Geometry check sheet. Reference: the model listing, model coordinates, mm. Face numbers are marked on the shaded views. A direction names the side the tool comes from. Round coordinates to 2 decimals unless told otherwise and drop trailing zeros. Loops run counter-clockwise (first coordinate to the right, second up) from the corner with the lowest first, then second, coordinate; pieces in that order, holes last. Notation, with made-up numbers: (11, 39) -> (47, 39) arc R24 ccw to (47, 77) -> close; hole circle Ø5 at (72, 63). An arc over 180 degrees is marked (long way). Use a Markdown table: item, result. Add a question column.
Q1. Sectioned sample at A-A, the plane x = 0. Enter the section's corners in (y, z), then the cut area to 3 significant figures.
Q2. Gauge pin test, flat ends, axial feed: P1, Ø2, axis at y = 35, z = 11.5, coming from the +X side; P2, Ø6, axis at x = 20, y = 0, coming from the +Z side; P3, Ø6, axis at y = -29, z = 10, coming from the +X side; P4, Ø3, axis at x = -20, y = 0, coming from the -Z side. Record the tip position at first contact, or that the pin passes through.
Q3. Material ranges on L1, parallel to Y at x = 0, z = 16; L2, parallel to Y at x = 0, z = 3.5; L3, parallel to Y at x = -1, z = 25.5, recorded low to high.
Q4. Sectioned sample at C-C, the plane y = 40. Enter the section's corners in (x, z), then the cut area to 4 significant figures.
Q5. Release check for a two-part mould opening along X. For the marked faces 3, 4 and 5 record: released by +X, released by -X, zero draft, split by the parting line, or undercut.
Q6. Sectioned sample at B-B, the plane y = 0. Enter the section's corners in (x, z), then the cut area to 3 significant figures.
Q7. Set-up check for the marked faces 1 and 2: record each of +Z, -Z, +X, -X, +Y, -Y from which the full face is reachable in a straight line by a thin tool's end or side.
Q8. Sectioned sample at D-D, the plane x = 20. Enter the section's corners in (y, z), then the cut area to 3 significant figures.
```python
from build123d import *

# Parameters (mm, degrees)
SKETCH1_R           = 50
SKETCH1_R_2         = 16
BOSS_EXTRUDE1_DEPTH = 8
SKETCH2_R           = 50
SKETCH2_R_2         = 30
BOSS_EXTRUDE2_DEPTH = 37
SKETCH3_R           = 2.5
CUT_EXTRUDE1_DEPTH  = 46
SKETCH4_R           = 2.5
CUT_EXTRUDE2_DEPTH  = 9


with BuildPart() as part:
    # Sketch1 → Boss-Extrude1 (new body)
    with BuildSketch(Plane.XY):
        Circle(SKETCH1_R)
        Circle(SKETCH1_R_2, mode=Mode.SUBTRACT)
    extrude(amount=BOSS_EXTRUDE1_DEPTH)

    # Sketch2 → Boss-Extrude2 (add)
    with BuildSketch(Plane.XY.offset(8)):
        Circle(SKETCH2_R)
        Circle(SKETCH2_R_2, mode=Mode.SUBTRACT)
    extrude(amount=BOSS_EXTRUDE2_DEPTH)

    # Sketch3 → Cut-Extrude1 (cut, through all)
    with BuildSketch(Plane.XY.offset(45)):
        with Locations((0, 40)):
            Circle(SKETCH3_R)
        with Locations((34.641016151, -20)):
            Circle(SKETCH3_R)
        with Locations((-34.641016151, -20)):
            Circle(SKETCH3_R)
    extrude(amount=-CUT_EXTRUDE1_DEPTH, mode=Mode.SUBTRACT)

    # Sketch4 → Cut-Extrude2 (cut, through all)
    with BuildSketch(Plane.XY.offset(8)):
        with Locations((0, 20)):
            Circle(SKETCH4_R)
        with Locations((20, 0)):
            Circle(SKETCH4_R)
        with Locations((0, -20)):
            Circle(SKETCH4_R)
        with Locations((-20, 0)):
            Circle(SKETCH4_R)
    extrude(amount=-CUT_EXTRUDE2_DEPTH, mode=Mode.SUBTRACT)


solid = part.part
```
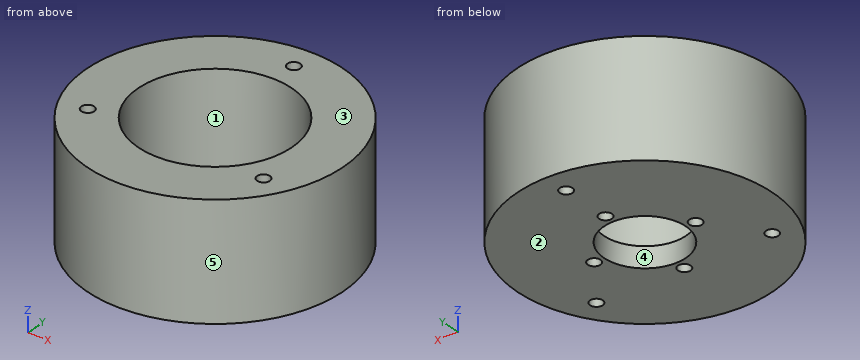
Values:
| question | item | result |
|---|---|---|
| 1 | outline | (-50, 0) -> (-22.5, 0) -> (-22.5, 8) -> (-30, 8) -> (-30, 45) -> (-50, 45) -> close; (-17.5, 0) -> (-16, 0) -> (-16, 8) -> (-17.5, 8) -> close; (16, 0) -> (17.5, 0) -> (17.5, 8) -> (16, 8) -> close; (22.5, 0) -> (37.5, 0) -> (37.5, 45) -> (30, 45) -> (30, 8) -> (22.5, 8) -> close; (42.5, 0) -> (50, 0) -> (50, 45) -> (42.5, 45) -> close |
| 1 | area | 1,720 mm^2 |
| 2 | P1 | x = 36.66 |
| 2 | P2 | z = 8 |
| 2 | P3 | x = 42.71 |
| 2 | P4 | through |
| 3 | L1 | -50 to -30, 30 to 37.5, 42.5 to 50 |
| 3 | L2 | -50 to -22.5, -17.5 to -16, 16 to 17.5, 22.5 to 37.5, 42.5 to 50 |
| 3 | L3 | -49.99 to -29.98, 29.98 to 37.71, 42.29 to 49.99 |
| 4 | outline | (-30, 0) -> (-2.5, 0) -> (-2.5, 45) -> (-30, 45) -> close; (2.5, 0) -> (30, 0) -> (30, 45) -> (2.5, 45) -> close |
| 4 | area | 2,475 mm^2 |
| 5 | face 3 | zero draft |
| 5 | face 4 | undercut |
| 5 | face 5 | split by the parting line |
| 6 | outline | (-50, 0) -> (-22.5, 0) -> (-22.5, 8) -> (-30, 8) -> (-30, 45) -> (-50, 45) -> close; (-17.5, 0) -> (-16, 0) -> (-16, 8) -> (-17.5, 8) -> close; (16, 0) -> (17.5, 0) -> (17.5, 8) -> (16, 8) -> close; (22.5, 0) -> (50, 0) -> (50, 45) -> (30, 45) -> (30, 8) -> (22.5, 8) -> close |
| 6 | area | 1,940 mm^2 |
| 7 | face 1 | +Z |
| 7 | face 2 | -Z, +X, -X, +Y, -Y |
| 8 | outline | (-45.83, 0) -> (-2.5, 0) -> (-2.5, 8) -> (-22.36, 8) -> (-22.36, 45) -> (-45.83, 45) -> close; (2.5, 0) -> (45.83, 0) -> (45.83, 45) -> (22.36, 45) -> (22.36, 8) -> (2.5, 8) -> close |
| 8 | area | 2,430 mm^2 |
